```python
from build123d import *

# Parameters (mm, degrees)
SKETCH1_W           = 225
SKETCH1_H           = 200
BOSS_EXTRUDE1_DEPTH = 3
CUT_EXTRUDE1_DEPTH  = 1
SKETCH4_R           = 4.9
BOSS_EXTRUDE2_DEPTH = 10
SKETCH5_W           = 150
SKETCH5_H           = 200
CUT_EXTRUDE2_DEPTH  = 10


with BuildPart() as part:
    # Sketch1 → Boss-Extrude1 (new body)
    with BuildSketch(Plane.XY):
        with Locations((112.5, 100)):
            Rectangle(SKETCH1_W, SKETCH1_H)
    extrude(amount=BOSS_EXTRUDE1_DEPTH)

    # Sketch2 → Cut-Extrude1 (cut)
    with BuildSketch(Plane.XY.offset(3)):
        Polygon((21.176597363, 159.100101172), (43.100604044, 183.764608689), (48.332469275, 179.114061817), (26.408462593, 154.4495543), align=None)
        Polygon((9.218048264, 169.729922593), (31.142054945, 194.39443011), (36.373920176, 189.743883238), (14.449913495, 165.079375722), align=None)
        Polygon((33.135146462, 148.470279751), (55.059153143, 173.134787267), (60.291018374, 168.484240396), (38.367011692, 143.819732879), align=None)
        Polygon((45.093695561, 137.840458329), (67.017702242, 162.504965846), (72.249567473, 157.854418974), (50.325560791, 133.189911458), align=None)
        Polygon((57.05224466, 127.210636908), (78.976251341, 151.875144425), (84.208116572, 147.224597553), (62.28410989, 122.560090036), align=None)
        Polygon((69.010793758, 116.580815487), (90.93480044, 141.245323003), (96.166665671, 136.594776132), (74.242658989, 111.930268615), align=None)
        Polygon((80.969342857, 105.950994066), (102.893349539, 130.615501582), (108.12521477, 125.96495471), (86.201208088, 101.300447194), align=None)
        Polygon((116.844990154, 74.061529802), (138.768996836, 98.726037318), (144.000862066, 94.075490447), (122.076855385, 69.41098293), align=None)
        Polygon((128.803539253, 63.431708381), (150.727545935, 88.096215897), (155.959411165, 83.445669025), (134.035404484, 58.781161509), align=None)
        Polygon((140.762088352, 52.801886959), (162.686095033, 77.466394476), (167.917960264, 72.815847604), (145.993953583, 48.151340087), align=None)
        Polygon((152.720637451, 42.172065538), (174.644644132, 66.836573055), (179.876509363, 62.186026183), (157.952502682, 37.521518666), align=None)
        Polygon((164.67918655, 31.542244117), (186.603193231, 56.206751633), (191.835058462, 51.556204761), (169.911051781, 26.891697245), align=None)
        Polygon((176.637735649, 20.912422695), (198.56174233, 45.576930212), (203.793607561, 40.92638334), (181.86960088, 16.261875824), align=None)
        Polygon((188.596284748, 10.282601274), (210.520291429, 34.947108791), (215.75215666, 30.296561919), (193.828149979, 5.632054402), align=None)
        Polygon((198.591537407, 154.4495543), (176.667530725, 179.114061817), (181.899395956, 183.764608689), (203.823402637, 159.100101172), align=None)
        Polygon((210.550086505, 165.079375721), (188.626079824, 189.743883238), (193.857945055, 194.39443011), (215.781951736, 169.729922593), align=None)
        Polygon((186.632988308, 143.819732879), (164.708981626, 168.484240395), (169.940846857, 173.134787267), (191.864853538, 148.470279751), align=None)
        Polygon((174.674439209, 133.189911458), (152.750432527, 157.854418974), (157.982297758, 162.504965846), (179.906304439, 137.840458329), align=None)
        Polygon((162.71589011, 122.560090036), (140.791883428, 147.224597553), (146.023748659, 151.875144425), (167.94775534, 127.210636908), align=None)
        Polygon((150.757341011, 111.930268615), (128.833334329, 136.594776132), (134.06519956, 141.245323003), (155.989206242, 116.580815487), align=None)
        Polygon((138.798791912, 101.300447194), (116.87478523, 125.96495471), (122.106650461, 130.615501582), (144.030657143, 105.950994066), align=None)
        Polygon((102.923144615, 69.41098293), (80.999137934, 94.075490447), (86.231003164, 98.726037318), (108.155009846, 74.061529802), align=None)
        Polygon((90.964595516, 58.781161509), (69.040588835, 83.445669025), (74.272454065, 88.096215897), (96.196460747, 63.431708381), align=None)
        Polygon((79.006046417, 48.151340087), (57.082039736, 72.815847604), (62.313904967, 77.466394476), (84.237911648, 52.801886959), align=None)
        Polygon((67.047497318, 37.521518666), (45.123490637, 62.186026183), (50.355355868, 66.836573055), (72.279362549, 42.172065538), align=None)
        Polygon((55.088948219, 26.891697245), (33.164941538, 51.556204761), (38.396806769, 56.206751633), (60.32081345, 31.542244117), align=None)
        Polygon((43.13039912, 16.261875824), (21.206392439, 40.92638334), (26.43825767, 45.576930212), (48.362264351, 20.912422695), align=None)
        Polygon((31.171850021, 5.632054402), (9.24784334, 30.296561919), (14.479708571, 34.947108791), (36.403715252, 10.282601274), align=None)
    extrude(amount=-CUT_EXTRUDE1_DEPTH, mode=Mode.SUBTRACT)

    # Sketch4 → Boss-Extrude2 (add)
    with BuildSketch(Plane(origin=(0, 0, 0), x_dir=(-1, 0, 0), z_dir=(0, 0, -1))):
        with Locations((-42.5, 190)):
            Circle(SKETCH4_R)
        with Locations((-22.5, 10)):
            Circle(SKETCH4_R)
    extrude(amount=BOSS_EXTRUDE2_DEPTH)

    # Sketch5 → Cut-Extrude2 (cut)
    with BuildSketch(Plane(origin=(0, 0, 0), x_dir=(-1, 0, 0), z_dir=(0, 0, -1))):
        with Locations((-150, 100)):
            Rectangle(SKETCH5_W, SKETCH5_H)
    extrude(amount=-CUT_EXTRUDE2_DEPTH, mode=Mode.SUBTRACT)


solid = part.part
```
Geometry check sheet. Reference: the model listing, model coordinates, mm. A direction names the side the tool comes from. Give positions to 0.01 mm unless a question says otherwise; leave off trailing zeros. Loops run counter-clockwise (first coordinate to the right, second up) from the corner with the lowest first, then second, coordinate; pieces in that order, holes last. Notation, with made-up numbers: (39.5, 37.25) - (78.5, 37.25) arc R23 ccw to (78.5, 75.25) - close; hole circle Ø4 at (-5.75, 17.25). An arc over 180 degrees is marked (long way). Use CSV: the item, a comma, the result in double quotes. Start each with the question number.
Q1. Go/stop test with flat-tipped pins: pin 1 Ø22.5 at (x, y) = (35, 106) entering from -Z; pin 2 Ø1.8 at (x, y) = (72.5, 116.5) entering from +Z; pin 3 Ø4 at (x, z) = (39.5, -3) entering from +Y. Record where each tip stops, or that it passes through.
Q2. Section check A-A, the plane z = -7.75. Record the cut outline in (x, y).
Q3. Release check for a two-part mould opening along Y. For faces 3 (the face through (43, 190, -10)), 4 (the face through (26.39, 7.02, -4.93)), 5 (the face through (35, 168, 2)) record: +Y half, -Y half, draft (parallel to the pull), parting line (faces both ways), or undercut.
Q4. Access from +Z, -Z, +X, -X, +Y, -Y to the whole of each face (thin tool, end or side, straight path). Record for faces 1 (the face through (59.705, 124.853, 2.507)), 2 (the face through (37, 101, 3)).
Q5. Scan lines: probe 1 along Z at (x, y) = (42.5, 98); probe 2 along Y at (x, z) = (43, -2.25); probe 3 along Z at (x, y) = (21, 26). Record each from-to range of solid material in increasing order. Write a range as from..to.
Findings below:
1,pin 1,"stops at z = 0"
1,pin 2,"stops at z = 2"
1,pin 3,"stops at y = 194.8"
2,outline,"circle Ø9.8 at (22.5, 10); circle Ø9.8 at (42.5, 190)"
3,face 3,"draft"
3,face 4,"parting line"
3,face 5,"undercut"
4,face 1,"+Z"
4,face 2,"+Z, +X, -X, +Y, -Y"
5,probe 1,"z = 0..3"
5,probe 2,"y = 185.13..194.87"
5,probe 3,"z = 0..2"
